Geometry check sheet. Reference: the model listing, model coordinates, mm. Give positions to 0.01 mm unless a question says otherwise; leave off trailing zeros. Order: outer loops, then holes, each group sorted by start corner. A loop starts at its lowest first (then second) coordinate and runs counter-clockwise, first axis right, second up. Notation, with made-up numbers: M -17,59.25 L 15,59.25 A30 cw 15,81.25 Z; hole C 50.25,71 d11. An arc over 180 degrees is marked long. Answer as CSV lines item,"result".
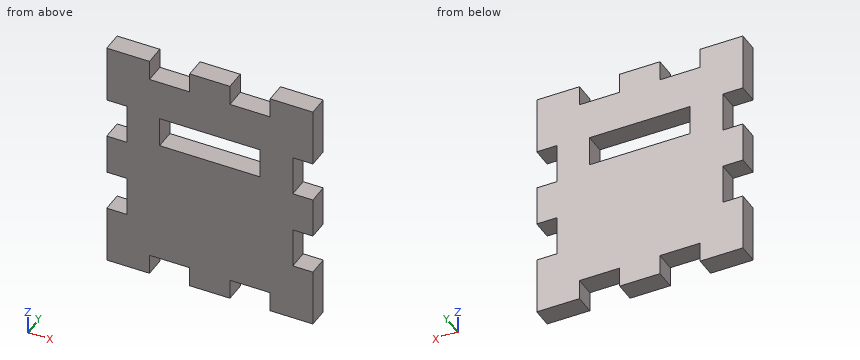
Autodesk Inventor part; units mm, degrees
ref_plane "YZ Plane" through (0, 0, 0) normal (1, 0, 0) x (0, 1, 0)
ref_plane "XZ Plane" through (0, 0, 0) normal (0, 1, 0) x (-1, 0, 0)
ref_plane "XY Plane" through (0, 0, 0) normal (0, 0, 1) x (1, 0, 0)
sketch "Sketch1" plane through (0, 0, 0) normal (0, 1, 0) x (-1, 0, 0)
  line L0 (0, 0) -> (-41, 0)
  line L1 (-41, 0) -> (-41, -47)
  line L2 (-41, -47) -> (0, -47)
  line L3 (0, -47) -> (0, 0)
  line L4 (-10.5, -18) -> (-30.5, -18)
  line L5 (-30.5, -18) -> (-30.5, -12)
  line L6 (-30.5, -12) -> (-10.5, -12)
  line L7 (-10.5, -12) -> (-10.5, -18)
  dimension "d0" = 41
  dimension "d1" = 47
  dimension "d2" = 20
  dimension "d3" = 6
  dimension "d4" = 10.5
  dimension "d5" = 12
extrude "Extrusion1" add sketch "Sketch1" along normal blind 4
sketch "Sketch2" plane through (0, 4, 0) normal (0, 1, 0) x (1, 0, 0)
  line L0 (41, 47) -> (0, 47) construction
  line L1 (0, 47) -> (0, 0) construction
  line L2 (0, 0) -> (41, 0) construction
  line L3 (41, 0) -> (41, 47) construction
  line L4 (4, 4) -> (4, 43) construction
  line L5 (4, 43) -> (37, 43) construction
  line L6 (37, 43) -> (37, 4) construction
  line L7 (37, 4) -> (4, 4) construction
  line L8 (0, 35.5) -> (4, 35.5)
  line L9 (4, 35.5) -> (4, 27.5)
  line L10 (4, 27.5) -> (0, 27.5)
  line L11 (0, 35.5) -> (0, 27.5)
  line L12 (0, 23.5) -> (41, 23.5) construction
  line L13 (20.5, 0) -> (20.5, 47) construction
  line L14 (41, 47) -> (0, 47) construction
  line L15 (8.5, 47) -> (8.5, 43)
  line L16 (8.5, 43) -> (16.5, 43)
  line L17 (16.5, 43) -> (16.5, 47)
  line L18 (16.5, 47) -> (8.5, 47)
  line L19 (41, 35.5) -> (37, 35.5)
  line L20 (37, 35.5) -> (37, 27.5)
  line L21 (37, 27.5) -> (41, 27.5)
  line L22 (41, 35.5) -> (41, 27.5)
  line L23 (32.5, 47) -> (32.5, 43)
  line L24 (32.5, 43) -> (24.5, 43)
  line L25 (24.5, 43) -> (24.5, 47)
  line L26 (24.5, 47) -> (32.5, 47)
  line L27 (41, 0) -> (0, 0)
  line L28 (4, 4) -> (37, 4)
  line L29 (0, 11.5) -> (4, 11.5)
  line L30 (4, 11.5) -> (4, 19.5)
  line L31 (4, 19.5) -> (0, 19.5)
  line L32 (0, 11.5) -> (0, 19.5)
  line L33 (41, 0) -> (0, 0)
  line L34 (8.5, 0) -> (8.5, 4)
  line L35 (8.5, 4) -> (16.5, 4)
  line L36 (16.5, 4) -> (16.5, 0)
  line L37 (16.5, 0) -> (8.5, 0)
  line L38 (24.5, 4) -> (24.5, 0)
  line L39 (32.5, 0) -> (32.5, 4)
  line L40 (37, 11.5) -> (37, 19.5)
  line L41 (41, 11.5) -> (37, 11.5)
  line L42 (41, 11.5) -> (41, 19.5)
  line L43 (37, 19.5) -> (41, 19.5)
  line L44 (24.5, 0) -> (32.5, 0)
  line L45 (32.5, 4) -> (24.5, 4)
  dimension "d8" = 4
  dimension "d9" = 8
  dimension "d10" = 4
  dimension "d11" = 8
  dimension "d12" = 4
extrude "Extrusion2" cut sketch "Sketch2" against normal up to surface (4 mm away) contours L8 L9 L10 L11 | L18 L17 L16 L15 | L22 L21 L20 L19 | L23 L24 L25 L26 | L27 L38 L28 L39 | L27 L34 L28 L36 | L32 L31 L30 L29 | L40 L43 L42 L41
properties part number "right" material "PBT Plastic Black"
(1) Section check B-B on z = -15. Enter the section's corners in (x, y), then the cut area to 3 significant figures.
The answers:
outline,"M 4,0 L 10.5,0 L 10.5,4 L 4,4 Z; M 30.5,0 L 37,0 L 37,4 L 30.5,4 Z"
area,"52.0 mm2"
(2) Section check A-A on x = 18.5. Enter the section's corners in (y, z), then the cut area to 3 significant figures.
The answers:
outline,"M 0,-47 L 4,-47 L 4,-18 L 0,-18 Z; M 0,-12 L 4,-12 L 4,0 L 0,0 Z"
area,"164 mm2"
(3) Material ranges on line 1 (X direction, y = 2.9, z = -3); line 2 (Z direction, x = 39.5, y = 2.2); line 3 (Z direction, x = 23, y = 1.4), recorded low to high.
The answers:
line 1,"x = 0 to 8.5, 16.5 to 24.5, 32.5 to 41"
line 2,"z = -47 to -35.5, -27.5 to -19.5, -11.5 to 0"
line 3,"z = -47 to -18, -12 to 0"
(4) Gauge pin test, flat ends, axial feed: P1, Ø4, axis at x = 17.5, z = -33.5, coming from the -Y side; P2, Ø2, axis at y = 2, z = -33, coming from the +X side; P3, Ø2, axis at y = 2, z = -17, coming from the -X side. Record the tip position at first contact, or that the pin passes through.
The answers:
P1,"stops at y = 0"
P2,"stops at x = 37"
P3,"stops at x = 4"
